Read the model definition and answer for the solid it produces. Units are mm, in the model's axes. Round coordinates to 2 decimals unless told otherwise and drop trailing zeros. Write each loop counter-clockwise with the first axis right and the second up, starting at its lowest first coordinate (ties: lowest second). Pieces come first, ordered by that corner, then holes. Notation, with made-up numbers: (-12, -22.75) -> (19, -22.75) arc R17 ccw to (19, -12.75) -> close; hole circle Ø8 at (67, 12.5). An arc over 180 degrees is marked (long way). Return JSON: item names as keys, results as strings. Group by question number.
(1) A cutting plane is placed at A-A on x = -5. Give the vertices of the cut face in (y, z).
(2) The mould has two halves that part along X. Classify faces 1 (the cylindrical face through (-6.9, 0.08, 2.47)), 2 (the flat face through (-11, 0, 2)), 3 (the flat face through (0, 6, 2)), 4 (the cylindrical face through (6.9, -0.08, 2.47)): released by +X, released by -X, zero draft, split by the parting line, or undercut.
(3) A cutting plane is placed at D-D on y = -1.25. State how many separate pieces and enclosed holes the cut face has, then the cut area to 3 significant figures.
(4) Straight lines are drawn through the part: line 1 (Y direction, x = 5, z = 1.4); line 2 (X direction, y = -1, z = 1.9); line 3 (X direction, y = -0.5, z = 1.55). For each, find the intervals that lie inside material, in ascending order.
(5) A cutting plane is placed at C-C on z = 3.4. Give the vertices of the cut face in (x, y).
(6) A cutting plane is placed at B-B on y = 0. Give the vertices of the cut face in (x, z), then the cut area to 3 significant figures.
```python
from build123d import *

# Parameters (mm, degrees)
SKETCH_1_W      = 22
SKETCH_1_H      = 12
SKETCH_1_R      = 1.9
EXTRUDE_1_DEPTH = 5
CHAMFER_1_SIZE  = 0.3


with BuildPart() as part:
    # 스케치1 → 보스-돌출1 (new body)
    with BuildSketch(Plane.XY):
        Rectangle(SKETCH_1_W, SKETCH_1_H)
        with Locations((-5, 0)):
            Circle(SKETCH_1_R, mode=Mode.SUBTRACT)
        with Locations(Location((5, 0, 0), (0, 0, 180))):
            Circle(SKETCH_1_R, mode=Mode.SUBTRACT)
    extrude(amount=EXTRUDE_1_DEPTH)

    # 모따기1
    chamfer_1_edges = [part.edges().sort_by_distance(p)[0] for p in [
        (-6.9, 0, 0),
        (-6.9, 0, 5),
        (-11, 0, 5),
        (6.9, 0, 0),
        (6.9, 0, 5),
        (0, -6, 5),
        (11, 0, 5),
        (0, -6, 0),
        (-11, 0, 0),
        (0, 6, 0),
        (11, 0, 0),
        (0, 6, 5),
    ]]
    chamfer(chamfer_1_edges, length=CHAMFER_1_SIZE)


solid = part.part
```
Checks:
{
 "1": {"outline": "(-6, 0.3) -> (-5.7, 0) -> (-2.2, 0) -> (-1.9, 0.3) -> (-1.9, 4.7) -> (-2.2, 5) -> (-5.7, 5) -> (-6, 4.7) -> close; (1.9, 0.3) -> (2.2, 0) -> (5.7, 0) -> (6, 0.3) -> (6, 4.7) -> (5.7, 5) -> (2.2, 5) -> (1.9, 4.7) -> close"},
 "2": {"face 1": "undercut", "face 2": "released by -X", "face 3": "zero draft", "face 4": "undercut"},
 "3": {"separate pieces": "3", "enclosed holes": "0", "area": "80.7 mm^2"},
 "4": {"line 1": "y = -6 to -1.9, 1.9 to 6", "line 2": "x = -11 to -6.62, -3.38 to 3.38, 6.62 to 11", "line 3": "x = -11 to -6.83, -3.17 to 3.17, 6.83 to 11"},
 "5": {"outline": "(-11, -6) -> (11, -6) -> (11, 6) -> (-11, 6) -> close; hole circle Ø3.8 at (-5, 0); hole circle Ø3.8 at (5, 0)"},
 "6": {"outline": "(-11, 0.3) -> (-10.7, 0) -> (-7.2, 0) -> (-6.9, 0.3) -> (-6.9, 4.7) -> (-7.2, 5) -> (-10.7, 5) -> (-11, 4.7) -> close; (-3.1, 0.3) -> (-2.8, 0) -> (2.8, 0) -> (3.1, 0.3) -> (3.1, 4.7) -> (2.8, 5) -> (-2.8, 5) -> (-3.1, 4.7) -> close; (6.9, 0.3) -> (7.2, 0) -> (10.7, 0) -> (11, 0.3) -> (11, 4.7) -> (10.7, 5) -> (7.2, 5) -> (6.9, 4.7) -> close", "area": "71.5 mm^2"}
}
